```python
from build123d import *

# Parameters (mm, degrees)
BOSS_EXTRUDE1_DEPTH     = 10
CUT_EXTRUDE1_DEPTH      = 72.414284285
CUT_EXTRUDE1_DEPTH_BACK = 72.414284285
SKETCH2_R               = 1.5
SKETCH9_W               = 10
SKETCH9_H               = 50
BOSS_EXTRUDE9_DEPTH     = 5
SKETCH10_W              = 10
SKETCH10_H              = 50
BOSS_EXTRUDE10_DEPTH    = 5
BOSS_EXTRUDE11_DEPTH    = 2
SKETCH12_W              = 10
SKETCH12_H              = 10
BOSS_EXTRUDE12_DEPTH    = 5
CUT_EXTRUDE2_START      = 7
SKETCH13_R              = 1.5
CUT_EXTRUDE2_DEPTH      = 7
BOSS_EXTRUDE13_DEPTH    = 2
SKETCH15_W              = 9.981523119
SKETCH15_H              = 10
BOSS_EXTRUDE14_DEPTH    = 30
SKETCH16_R              = 1.5
CUT_EXTRUDE3_DEPTH      = 32
SKETCH17_W              = 10
SKETCH17_H              = 89
BOSS_EXTRUDE15_DEPTH    = 30
SKETCH19_W              = 5
SKETCH19_H              = 89
BOSS_EXTRUDE16_DEPTH    = 15
FILLET1_R               = 5
SKETCH20_R              = 2
CUT_EXTRUDE4_DEPTH      = 149.657324071
SKETCH21_R              = 2
CUT_EXTRUDE5_DEPTH      = 10
SKETCH22_W              = 110
SKETCH22_H              = 89
CUT_EXTRUDE6_DEPTH      = 104.435970532


with BuildPart() as part:
    # Sketch1 → Boss-Extrude1 (new body)
    with BuildSketch(Plane.XY):
        with BuildLine():
            Line((45.018476881, -25), (50, -25))
            Line((50, -25), (50, 25))
            Line((50, 25), (45, 25))
            ThreePointArc((45, 25), (0, 8), (-45, 25))
            Line((-45, 25), (-50, 25))
            Line((-50, 25), (-50, -25))
            Line((-50, -25), (-45.018476881, -25))
            ThreePointArc((-45.018476881, -25), (0, -8), (45.018476881, -25))
        make_face()
    extrude(amount=BOSS_EXTRUDE1_DEPTH)

    # Sketch2 → Cut-Extrude1 (cut, two sides: drawn at the far end of the back side and taken through both)
    with BuildSketch(Plane(origin=(0, 25, 0), x_dir=(1, 0, 0), z_dir=(0, 1, 0)).offset(-CUT_EXTRUDE1_DEPTH_BACK)):
        with Locations(Location((-48, -5, 0), (0, 0, 180))):
            Circle(SKETCH2_R)
        with Locations(Location((48, -5, 0), (0, 0, 180))):
            Circle(SKETCH2_R)
    extrude(amount=CUT_EXTRUDE1_DEPTH + CUT_EXTRUDE1_DEPTH_BACK, mode=Mode.SUBTRACT)

    # Sketch9 → Boss-Extrude9 (add)
    with BuildSketch(Plane(origin=(50, 0, 0), x_dir=(0, 0, -1), z_dir=(1, 0, 0))):
        with Locations((-5, 0)):
            Rectangle(SKETCH9_W, SKETCH9_H)
    extrude(amount=BOSS_EXTRUDE9_DEPTH)

    # Sketch10 → Boss-Extrude10 (add)
    with BuildSketch(Plane.ZY.offset(50)):
        with Locations((5, 0)):
            Rectangle(SKETCH10_W, SKETCH10_H)
    extrude(amount=BOSS_EXTRUDE10_DEPTH)

    # Sketch11 → Boss-Extrude11 (add)
    with BuildSketch(Plane(origin=(0, 25, 0), x_dir=(1, 0, 0), z_dir=(0, 1, 0))):
        Polygon((50, 0), (50, -7), (45, -7), (45, -10), (55, -10), (55, 0), align=None)
        Polygon((-50, 0), (-50, -7), (-45, -7), (-45, -10), (-55, -10), (-55, 0), align=None)
    extrude(amount=BOSS_EXTRUDE11_DEPTH)

    # Sketch12 → Boss-Extrude12 (add)
    with BuildSketch(Plane(origin=(0, 27, 0), x_dir=(1, 0, 0), z_dir=(0, 1, 0))):
        with Locations((50, -5)):
            Rectangle(SKETCH12_W, SKETCH12_H)
        with Locations((-50, -5)):
            Rectangle(SKETCH12_W, SKETCH12_H)
    extrude(amount=BOSS_EXTRUDE12_DEPTH)

    # Sketch13 → Cut-Extrude2 (cut)
    with BuildSketch(Plane(origin=(0, 25, 0), x_dir=(1, 0, 0), z_dir=(0, 1, 0)).offset(CUT_EXTRUDE2_START)):
        with Locations(Location((48, -5, 0), (0, 0, 180))):
            Circle(SKETCH13_R)
        with Locations(Location((-48, -5, 0), (0, 0, 180))):
            Circle(SKETCH13_R)
    extrude(amount=-CUT_EXTRUDE2_DEPTH, mode=Mode.SUBTRACT)

    # Sketch14 → Boss-Extrude13 (add)
    with BuildSketch(Plane.XZ.offset(25)):
        Polygon((50.009238441, 0), (50.009238441, 7), (45.018476881, 7), (45.018476881, 10), (55, 10), (55, 0), align=None)
        Polygon((-50.009238441, 0), (-50.009238441, 7), (-45.018476881, 7), (-45.018476881, 10), (-55, 10), (-55, 0), align=None)
    extrude(amount=BOSS_EXTRUDE13_DEPTH)

    # Sketch15 → Boss-Extrude14 (add)
    with BuildSketch(Plane.XZ.offset(27)):
        with Locations((-50.00923844, 5)):
            Rectangle(SKETCH15_W, SKETCH15_H)
        with Locations((50.00923844, 5)):
            Rectangle(SKETCH15_W, SKETCH15_H)
    extrude(amount=BOSS_EXTRUDE14_DEPTH)

    # Sketch16 → Cut-Extrude3 (cut)
    with BuildSketch(Plane.XZ.offset(25)):
        with Locations(Location((48, 5, 0), (0, 0, 180))):
            Circle(SKETCH16_R)
        with Locations(Location((-48, 5, 0), (0, 0, 180))):
            Circle(SKETCH16_R)
    extrude(amount=CUT_EXTRUDE3_DEPTH, mode=Mode.SUBTRACT)

    # Sketch17 → Boss-Extrude15 (add)
    with BuildSketch(Plane.ZY.offset(55)):
        with Locations((5, -12.5)):
            Rectangle(SKETCH17_W, SKETCH17_H)
    extrude(amount=BOSS_EXTRUDE15_DEPTH)

    # Sketch19 → Boss-Extrude16 (add)
    with BuildSketch(Plane.XY.offset(10)):
        with Locations((-82.5, -12.5)):
            Rectangle(SKETCH19_W, SKETCH19_H)
    extrude(amount=BOSS_EXTRUDE16_DEPTH)

    # Fillet1
    fillet1_edges = [part.edges().sort_by_distance(p)[0] for p in [
        (-80, -12.5, 10),
    ]]
    fillet(fillet1_edges, radius=FILLET1_R)

    # Sketch20 → Cut-Extrude4 (cut, through all)
    with BuildSketch(Plane(origin=(-80, 0, 0), x_dir=(0, 0, -1), z_dir=(1, 0, 0))):
        with Locations(Location((-20, 9.75, 0), (0, 0, 90))):
            Circle(SKETCH20_R)
        with Locations(Location((-20, -12.5, 0), (0, 0, 90))):
            Circle(SKETCH20_R)
        with Locations(Location((-20, -34.75, 0), (0, 0, 90))):
            Circle(SKETCH20_R)
    extrude(amount=-CUT_EXTRUDE4_DEPTH, mode=Mode.SUBTRACT)

    # Sketch21 → Cut-Extrude5 (cut)
    with BuildSketch(Plane.XY.offset(10)):
        with Locations((-65, 20.875)):
            Circle(SKETCH21_R)
        with Locations((-65, -1.375)):
            Circle(SKETCH21_R)
        with Locations((-65, -23.625)):
            Circle(SKETCH21_R)
        with Locations((-65, -45.875)):
            Circle(SKETCH21_R)
    extrude(amount=-CUT_EXTRUDE5_DEPTH, mode=Mode.SUBTRACT)

    # Sketch22 → Cut-Extrude6 (cut, through all)
    with BuildSketch(Plane.XY.offset(10)):
        with Locations((0, -12.5)):
            Rectangle(SKETCH22_W, SKETCH22_H)
    extrude(amount=-CUT_EXTRUDE6_DEPTH, mode=Mode.SUBTRACT)


solid = part.part
```
Geometry check sheet. Reference: the model listing, model coordinates, mm. A direction names the side the tool comes from. Give positions to 0.01 mm unless a question says otherwise; leave off trailing zeros. Order: outer loops, then holes, each group sorted by start corner. A loop starts at its lowest first (then second) coordinate and runs counter-clockwise, first axis right, second up.
1. Section check C-C, the plane y = -39.5. Enter the section's corners in (x, z), and give its area (3 significant figures).
2. Section check A-A, the plane y = 9.75. Enter the section's corners in (x, z), and give its area (3 significant figures).
3. Gauge pin test, flat ends, axial feed: pin 1 Ø4 at (x, y) = (-66.5, -27) entering from +Z; pin 2 Ø5 at (y, z) = (-34.75, 20) entering from -X; pin 3 Ø3 at (y, z) = (-7, 21.5) entering from +X; pin 4 Ø1 at (y, z) = (9.5, 12) entering from +X. Record the tip position at first contact, or that the pin passes through.
4. Access from +Z, -Z, +X, -X, +Y, -Y to the whole of each face (thin tool, end or side, straight path). Record for faces 1 (the face through (-65, -13, 10)), 2 (the face through (-66.5, -22.3, 5.1)).
5. Thickness scan on L1, parallel to Y at x = -65, z = 7 (3 decimals); L2, parallel to X at y = 21, z = 9.25; L3, parallel to Z at x = -73, y = 7. Record the ranges inside material, lowest first.
6. Release check for a two-part mould opening along Z. For faces 3 (the face through (-82.465, 9.49, 21.983)), 4 (the face through (-70, -13, 0)), 5 (the face through (-66.5, 22.2, 5.1)), 6 (the face through (-82.465, -12.76, 21.983)) record: pulls with the +Z half, pulls with the -Z half, needs draft (parallel to the pull), parting line crosses it, or undercut.
7. Section check B-B, the plane x = -65. Enter the section's corners in (y, z) (3 decimals), and give its area (3 significant figures).
Values follow:
1. outline: (-85, 0) - (-55, 0) - (-55, 10) - (-75, 10) arc R5 cw to (-80, 15) - (-80, 25) - (-85, 25) - close
1. area: 380 mm2
2. outline: (-85, 0) - (-55, 0) - (-55, 10) - (-75, 10) arc R5 cw to (-80, 15) - (-80, 18) - (-85, 18) - close; (-85, 22) - (-80, 22) - (-80, 25) - (-85, 25) - close
2. area: 360 mm2
3. pin 1: stops at z = 10
3. pin 2: stops at x = -85
3. pin 3: stops at x = -80
3. pin 4: stops at x = -78.57
4. face 1: +Z, +X, +Y, -Y
4. face 2: +Z, -Z
5. L1: y = -57 to -47.875, -43.875 to -25.625, -21.625 to -3.375, 0.625 to 18.875, 22.875 to 32
5. L2: x = -85 to -67, -63 to -55
5. L3: z = 0 to 10
6. face 3: undercut
6. face 4: pulls with the -Z half
6. face 5: needs draft
6. face 6: undercut
7. outline: (-57, 0) - (-47.875, 0) - (-47.875, 10) - (-57, 10) - close; (-43.875, 0) - (-25.625, 0) - (-25.625, 10) - (-43.875, 10) - close; (-21.625, 0) - (-3.375, 0) - (-3.375, 10) - (-21.625, 10) - close; (0.625, 0) - (18.875, 0) - (18.875, 10) - (0.625, 10) - close; (22.875, 0) - (32, 0) - (32, 10) - (22.875, 10) - close
7. area: 730 mm2
